Build history of the part. All positions in model axes, mm. A direction names the side the tool comes from. Give positions to 0.01 mm unless a question says otherwise; leave off trailing zeros. Loops run counter-clockwise (first coordinate to the right, second up) from the corner with the lowest first, then second, coordinate; pieces in that order, holes last. Notation, with made-up numbers: M -6.5,37 L 47.5,37 A19 cw 47.5,66 Z; hole C 19.25,34.25 d2. An arc over 180 degrees is marked long. Put each result on its own line as item: value.
Autodesk Inventor part; units mm, degrees
ref_plane "YZ Plane" through (0, 0, 0) normal (1, 0, 0) x (0, 1, 0)
ref_plane "XZ Plane" through (0, 0, 0) normal (0, 1, 0) x (-1, 0, 0)
ref_plane "XY Plane" through (0, 0, 0) normal (0, 0, 1) x (1, 0, 0)
sketch "スケッチ1" plane through (0, 0, 0) normal (0, 0, 1) x (1, 0, 0)
  line L0 (-15, -45) -> (15, -45)
  line L1 (15, -45) -> (15, 45)
  line L2 (15, 45) -> (-15, 45)
  line L3 (-15, 45) -> (-15, -45)
  point P0 (0, 0)
  point P1 (0, -45)
  point P2 (-15, 0)
  dimension "d0" = 30
  dimension "d1" = 90
extrude "押し出し1" add sketch "スケッチ1" along normal blind 15
sketch "スケッチ6" plane through (0, 0, 15) normal (0, 0, 1) x (1, 0, 0)
  line L0 (15, -45) -> (-15, -45)
  point P0 (0, 0)
  point P1 (-11, -40)
  dimension "d33" = 11
  dimension "d52" = 5
hole "穴3" at (-11, -40, 15) direction (0, 0, -1) diameter 3.242 end through all
pattern_linear "矩形状パターン2" count 2 spacing 22 along (1, 0, 0) count 2 spacing 46 along (0, 1, 0) of "穴3"
sketch "スケッチ9" plane through (0, 0, 15) normal (0, 0, 1) x (1, 0, 0)
  line L0 (15, -45) -> (-15, -45)
  point P0 (0, 0)
  point P1 (-10, -18)
  point P2 (10, -18)
  dimension "d53" = 27
  dimension "d54" = 10
  dimension "d62" = 10
hole "穴4" at (-10, -18, 15) at (10, -18, 15) direction (0, 0, -1) diameter 4.5 end through all counterbore diameter 8 counterbore depth 4.5
sketch "スケッチ10" plane through (0, 0, 15) normal (0, 0, 1) x (1, 0, 0)
  circle A0 centre (-11, 6) radius 1.621
  line L0 (-15, -45) -> (-15, 45)
  line L1 (15, 45) -> (15, -45)
  line L2 (-15, 45) -> (15, 45)
  line L3 (-15, 11) -> (15, 11)
  point P0 (0, 0)
  dimension "d63" = 5
extrude "押し出し5" cut sketch "スケッチ10" against normal blind 7.1 contours L0 L2 L1 L3
sketch "スケッチ11" plane through (0, 0, 7.9) normal (0, 0, 1) x (1, 0, 0)
  circle A0 centre (-10, -18) radius 4
  circle A1 centre (10, -18) radius 4
  point P0 (0, 0)
  point P1 (-10, 16)
  point P2 (10, 16)
  dimension "d66" = 34
hole "穴5" at (-10, 16, 7.9) at (10, 16, 7.9) direction (0, 0, -1) diameter 4.5 end through all counterbore diameter 8 counterbore depth 4.5
chamfer "面取り1" distance 1 angle 45 2 edges at (15, 45, 3.95) (-15, 45, 3.95)
sketch "スケッチ12" plane through (0, 0, 0) normal (0, 0, -1) x (-1, 0, 0)
  line L0 (15, -45) -> (-15, -45)
  circle A0 centre (-10, 16) radius 2.25
  circle A1 centre (-10, -18) radius 2.25
  point P0 (0, 0)
  point P1 (0, 16)
  point P2 (0, -18)
  point P3 (0, -45)
hole "穴6" at (0, 16, 0) at (0, -18, 0) direction (0, 0, 1) diameter 4 depth 8 tip angle 118
chamfer "面取り2" distance 2 angle 45 1 edges at (0, -45, 0)
properties part number "04" material "A5052"
Q1. Tool access for faces 1 (the flat face through (0, 28, 7.9)), 2 (the cylindrical face through (12.4, -14.8, 12.7)), 3 (the cylindrical face through (-12.607, 6.211, 7.395)): list every direction of +Z, -Z, +X, -X, +Y, -Y with a clear straight run to the whole face (end or side of a thin tool).
Here are the results:
face 1: +Z, +X, -X, +Y
face 2: +Z
face 3: +Z, -Z
Q2. Slice it at A-A (y = 6). List the corners of the cut face in (x, z), and give its area (3 significant figures).
Here are the results:
outline: M -15,0 L -12.62,0 L -12.62,15 L -15,15 Z; M -9.38,0 L 9.38,0 L 9.38,15 L -9.38,15 Z; M 12.62,0 L 15,0 L 15,15 L 12.62,15 Z
area: 353 mm²
Q3. Slice it at C-C (y = 16). List the corners of the cut face in (x, z), and give its area (3 significant figures).
Here are the results:
outline: M -15,0 L -12.25,0 L -12.25,3.4 L -14,3.4 L -14,7.9 L -15,7.9 Z; M -7.75,0 L -2,0 L -2,7.9 L -6,7.9 L -6,3.4 L -7.75,3.4 Z; M 2,0 L 7.75,0 L 7.75,3.4 L 6,3.4 L 6,7.9 L 2,7.9 Z; M 12.25,0 L 15,0 L 15,7.9 L 14,7.9 L 14,3.4 L 12.25,3.4 Z
area: 103 mm²
Q4. Drop flat-ended pins along their axis: pin 1 Ø7 at (x, y) = (-10, -18) entering from -Z; pin 2 Ø5 at (x, y) = (10, 16) entering from +Z; pin 3 Ø6.5 at (x, y) = (12, 15) entering from +Z; pin 4 Ø3 at (x, y) = (0, -18) entering from -Z. Give the stop position or say it passes through.
Here are the results:
pin 1: z = 0
pin 2: z = 3.4
pin 3: z = 7.9
pin 4: z = 8.3
Q5. Slice it at B-B (z = 6.5). State how many separate pieces and enclosed holes the cut face has, and give its area (3 significant figures).
Here are the results:
separate pieces: 1
enclosed holes: 10
area: 2,510 mm²
Q6. Probe line 1 (X direction, y = 16, z = 6.05); line 2 (Y direction, x = -11, z = 10); line 3 (X direction, y = -18, z = 7.25). List the from-to ranges inside material, lowest first. Write a range as from..to.
Here are the results:
line 1: -15..-14, -6..-2, 2..6, 14..15
line 2: -45..-41.62, -38.38..-20.02, -15.98..4.38, 7.62..11
line 3: -15..-12.25, -7.75..-2, 2..7.75, 12.25..15
Q7. Mould opens along X. For faces 4 (the flat face through (-15, -10, 7)), 5 (the flat face through (0, -44, 1)), 6 (the flat face through (-8, -20, 10.5)) say: pulls with the +X half, pulls with the -X half, needs draft (parallel to the pull), parting line crosses it, or undercut.
Here are the results:
face 4: pulls with the -X half
face 5: needs draft
face 6: undercut
Q8. Slice it at D-D (x = 5). List the corners of the cut face in (y, z).
Here are the results:
outline: M -45,2 L -43,0 L 45,0 L 45,7.9 L 11,7.9 L 11,15 L -45,15 Z
